Check sheet for the modelled part. Datum: model origin and axes. Units: mm. A direction names the side the tool comes from. Round coordinates to 2 decimals unless told otherwise and drop trailing zeros. Loops run counter-clockwise (first coordinate to the right, second up) from the corner with the lowest first, then second, coordinate; pieces in that order, holes last. Notation, with made-up numbers: (-20, -37) -> (16, -37) arc R21 cw to (16, -15) -> close; hole circle Ø5 at (74.5, -6.5). An arc over 180 degrees is marked (long way). Use one line per item in the form item = value. Start each with the question number.
(1) Set-up check for faces 1 (the flat face through (-18.03, -20, 18)), 2 (the flat face through (-13, -20, -13.764)), 3 (the flat face through (-3.809, -20, 0)): record each of +Z, -Z, +X, -X, +Y, -Y from which the full face is reachable in a straight line by a thin tool's end or side.
(2) Material ranges on probe 1 along X at (y, z) = (-21, -19.5); probe 2 along X at (y, z) = (-11, 24); probe 3 along Z at (x, y) = (-14.5, -27), recorded low to high. Write a range as [from, to].
(3) Go/stop test with flat-tipped pins: pin 1 (3 mm diameter, centred on x = -20, y = -11.5, fed in from -Z); pin 2 (14.5 mm diameter, centred on y = -15, z = 22, fed in from -X); pin 3 (2.5 mm diameter, centred on x = -13, y = -18.5, fed in from -Z); pin 4 (1 mm diameter, centred on x = -21, y = -13, fed in from +Z). Record where each tip stops, or that it passes through.
(4) Sectioned sample at D-D (z = 15). Record the cut outline in (x, y), and give its area (3 significant figures).
(5) Sectioned sample at A-A (z = -18). Record the cut outline in (x, y), and give its area (3 significant figures).
(6) Sectioned sample at C-C (x = -13.25). Record the cut outline in (y, z), and give its area (3 significant figures).
(7) Draft check along X on faces 4 (the flat face through (-14, 0, 0)), 5 (the flat face through (-13, -20, 13.764)), 6 (the cylindrical face through (-7.09, -19.72, -31.05)), 7 (the cylindrical face through (-17.3, -20.3, -14.5)). Enter one of: released by +X, released by -X, zero draft, split by the parting line, or undercut.
(8) Sectioned sample at B-B (y = -7.5). Record the cut outline in (x, z), and give its area (3 significant figures).
from build123d import *

# Parameters (mm, degrees)
F1_DEPTH    = 40
F2_R        = 2.5
F3_T1_DEPTH = 50


# Not quite as in the source:
# - a fillet or chamfer that OpenCascade refuses, or shapes differently, is made with other operations: its cross-section is extruded or revolved along the edge and cut away or added


with BuildPart() as f1:
    # F0 (on Front) → F1 (new body)
    with BuildSketch(Plane.XZ):
        Polygon((-23.9221176861, 22.5), (-23.9221176861, 0), (-23.9221176861, -22.5), (-18.0304694658, -22.5), (-18.0304694658, -13.7641071746), (-7.6692953279, -13.7641071746), (-7.6692953279, -31.6422108453), (-3.809250768, -31.6422108453), (-3.809250768, 0), (-3.809250768, 31.6422108453), (-7.6692953279, 31.6422108453), (-7.6692953279, 13.7641071746), (-18.0304694658, 13.7641071746), (-18.0304694658, 22.5), align=None)
    extrude(amount=F1_DEPTH)

    # F2
    f2_edges = [f1.edges().sort_by_distance(p)[0] for p in [
        (-23.922118, -20, 22.5),
        (-18.030469, -20, 22.5),
        (-23.922118, -20, -22.5),
        (-18.030469, -20, -22.5),
        (-18.030469, -20, 13.764107),
        (-18.030469, -20, -13.764107),
        (-7.669295, -20, 13.764107),
        (-7.669295, -20, -13.764107),
    ]]
    fillet(f2_edges, radius=F2_R)

    # F3: fillet of radius 2 on 4 edges, made by hand

    # F3_s2 → F3_t1 (cut)
    with BuildSketch(Plane.XZ.offset(-5)):
        with BuildLine():
            ThreePointArc((-7.6692953279, 29.6422108453), (-7.0835088902, 31.0564244077), (-5.6692953279, 31.6422108453))
            Line((-5.6692953279, 31.6422108453), (-7.6692953279, 31.6422108453))
            Line((-7.6692953279, 31.6422108453), (-7.6692953279, 29.6422108453))
        make_face()
        with BuildLine():
            ThreePointArc((-5.809250768, 31.6422108453), (-4.3950372056, 31.0564244077), (-3.809250768, 29.6422108453))
            Line((-3.809250768, 29.6422108453), (-3.809250768, 31.6422108453))
            Line((-3.809250768, 31.6422108453), (-5.809250768, 31.6422108453))
        make_face()
        with BuildLine():
            ThreePointArc((-5.6692953279, -31.6422108453), (-7.0835088902, -31.0564244077), (-7.6692953279, -29.6422108453))
            Line((-7.6692953279, -29.6422108453), (-7.6692953279, -31.6422108453))
            Line((-7.6692953279, -31.6422108453), (-5.6692953279, -31.6422108453))
        make_face()
        with BuildLine():
            ThreePointArc((-3.809250768, -29.6422108453), (-4.3950372056, -31.0564244077), (-5.809250768, -31.6422108453))
            Line((-5.809250768, -31.6422108453), (-3.809250768, -31.6422108453))
            Line((-3.809250768, -31.6422108453), (-3.809250768, -29.6422108453))
        make_face()
    extrude(amount=F3_T1_DEPTH, mode=Mode.SUBTRACT)


solid = f1.part
Checks:
q1.face_1 = +Z, +Y, -Y
q1.face_2 = -Z, +Y, -Y
q1.face_3 = +Z, -Z, +X, +Y, -Y
q2.probe_1 = [-23.92, -18.03], [-7.67, -3.81]
q2.probe_2 = [-7.67, -3.81]
q2.probe_3 = [-13.76, 13.76]
q3.pin_1 = -22.5
q3.pin_2 = -23.92
q3.pin_3 = -13.76
q3.pin_4 = 22.5
q4.outline = (-23.92, -40) -> (-17.69, -40) -> (-17.69, 0) -> (-23.92, 0) -> close; (-8.01, -40) -> (-3.81, -40) -> (-3.81, 0) -> (-8.01, 0) -> close
q4.area = 418 mm2
q5.outline = (-23.92, -40) -> (-18.03, -40) -> (-18.03, 0) -> (-23.92, 0) -> close; (-7.67, -40) -> (-3.81, -40) -> (-3.81, 0) -> (-7.67, 0) -> close
q5.area = 390 mm2
q6.outline = (-40, -13.76) -> (0, -13.76) -> (0, 13.76) -> (-40, 13.76) -> close
q6.area = 1,100 mm2
q7.face_4 = zero draft
q7.face_5 = undercut
q7.face_6 = released by -X
q7.face_7 = undercut
q8.outline = (-23.92, -20) arc R2.5 ccw to (-21.42, -22.5) -> (-20.53, -22.5) arc R2.5 ccw to (-18.03, -20) -> (-18.03, -16.26) arc R2.5 cw to (-15.53, -13.76) -> (-10.17, -13.76) arc R2.5 cw to (-7.67, -16.26) -> (-7.67, -29.64) arc R2 ccw to (-5.74, -31.64) arc R2 ccw to (-3.81, -29.64) -> (-3.81, 29.64) arc R2 ccw to (-5.74, 31.64) arc R2 ccw to (-7.67, 29.64) -> (-7.67, 16.26) arc R2.5 cw to (-10.17, 13.76) -> (-15.53, 13.76) arc R2.5 cw to (-18.03, 16.26) -> (-18.03, 20) arc R2.5 ccw to (-20.53, 22.5) -> (-21.42, 22.5) arc R2.5 ccw to (-23.92, 20) -> close
q8.area = 791 mm2
